Part model, mm, in its own coordinate system. Face numbers are marked on the shaded views. A direction names the side the tool comes from. Round coordinates to 2 decimals unless told otherwise and drop trailing zeros. Loops run counter-clockwise (first coordinate to the right, second up) from the corner with the lowest first, then second, coordinate; pieces in that order, holes last. Notation, with made-up numbers: M 86.25,33 L 123.25,33 A9 ccw 123.25,46 Z; hole C 61.5,-24.75 d7. An arc over 180 degrees is marked long. Put each result on its own line as item: value. Start each with the question number.
```python
from build123d import *

# Parameters (mm, degrees)
SKETCH1_W           = 10
SKETCH1_H           = 25.2
BOSS_EXTRUDE1_DEPTH = 4
SKETCH2_W           = 10
SKETCH2_H           = 3.2
SKETCH2_H_2         = 7.7
BOSS_EXTRUDE2_DEPTH = 7
SKETCH3_W           = 10
SKETCH3_H           = 4.5
BOSS_EXTRUDE3_DEPTH = 13
SKETCH4_R           = 3.1
CUT_EXTRUDE2_DEPTH  = 1
CHAMFER2_SIZE       = 1
CHAMFER3_SIZE       = 3


with BuildPart() as part:
    # Sketch1 → Boss-Extrude1 (new body)
    with BuildSketch(Plane.XY):
        with Locations((5, 12.6)):
            Rectangle(SKETCH1_W, SKETCH1_H)
    extrude(amount=BOSS_EXTRUDE1_DEPTH)

    # Sketch2 → Boss-Extrude2 (add)
    with BuildSketch(Plane(origin=(0, 0, 0), x_dir=(-1, 0, 0), z_dir=(0, 0, -1))):
        with Locations((-5, 23.6)):
            Rectangle(SKETCH2_W, SKETCH2_H)
        with Locations((-5, 12.85)):
            Rectangle(SKETCH2_W, SKETCH2_H_2)
    extrude(amount=BOSS_EXTRUDE2_DEPTH)

    # Sketch3 → Boss-Extrude3 (add)
    with BuildSketch(Plane.XY.offset(4)):
        with Locations((5, 2.25)):
            Rectangle(SKETCH3_W, SKETCH3_H)
    extrude(amount=BOSS_EXTRUDE3_DEPTH)

    # Sketch4 → Cut-Extrude2 (cut)
    with BuildSketch(Plane(origin=(0, 4.5, 0), x_dir=(1, 0, 0), z_dir=(0, 1, 0))):
        with Locations(Location((5, -9, 0), (0, 0, 270))):
            Circle(SKETCH4_R)
    extrude(amount=-CUT_EXTRUDE2_DEPTH, mode=Mode.SUBTRACT)

    # Chamfer2
    chamfer2_edges = [part.edges().sort_by_distance(p)[0] for p in [
        (5, 3.5, 5.9),
    ]]
    chamfer(chamfer2_edges, length=CHAMFER2_SIZE - 0.0001)  # a hair under: the kernel refuses the full size

    # Chamfer3
    chamfer3_edges = [part.edges().sort_by_distance(p)[0] for p in [
        (5, 25.2, 4),
        (5, 4.5, 17),
    ]]
    chamfer(chamfer3_edges, length=CHAMFER3_SIZE)


solid = part.part
```
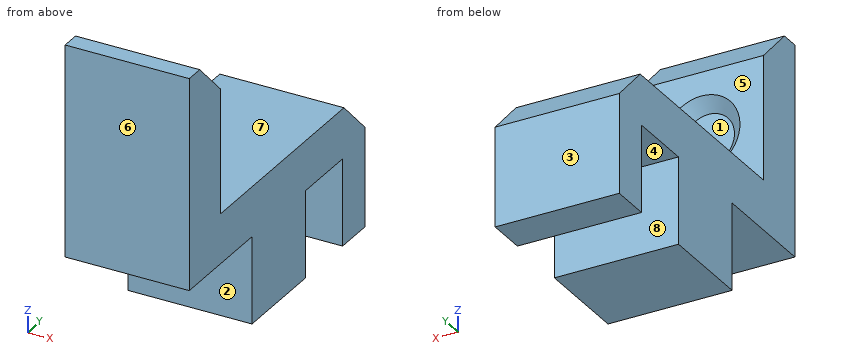
1. Wall check: L1, parallel to Y at x = 2, z = -4.75; L2, parallel to Y at x = 6.5, z = 9; L3, parallel to Z at x = 5, y = 4.55. Give the ranges that are in metal, low to high.
2. Mould opens along Y. For the marked faces 6, 7 and 8 say: released by +Y, released by -Y, zero draft, split by the parting line, or undercut.
3. Cut at D-D, the plane y = 2.25. Give the cut face in (x, z), and give its area (4 significant figures).
4. Drop flat-ended pins along their axis: pin 1 (4.5 mm diameter, centred on x = 4, z = 9, fed in from +Y); pin 2 (5 mm diameter, centred on x = 3.5, y = 17.5, fed in from +Z); pin 3 (2 mm diameter, centred on x = 4, z = -2.5, fed in from -Y). Give the stop position or say it passes through.
5. Which spindle directions (+Z, -Z, +X, -X, +Y, -Y) get a long thin tool onto all of the face, cutting with end or side? Do the marked faces 1, 2, 3, 4 and 5. Say none if no direction does.
6. Cut at A-A, the plane z = -3. Give the cut face in (x, y).
Results list:
1. L1: y = 9 to 16.7, 22 to 25.2
1. L2: y = 0 to 3.5
1. L3: z = 0 to 4
2. face 6: released by -Y
2. face 7: zero draft
2. face 8: undercut
3. outline: M 0,0 L 10,0 L 10,16.25 L 0,16.25 Z
3. area: 162.5 mm^2
4. pin 1: stops at y = 4.5
4. pin 2: stops at z = 4
4. pin 3: stops at y = 9
5. face 1: +Y
5. face 2: -Z, +X, -X, -Y
5. face 3: +Z, -Z, +X, -X, +Y
5. face 4: -Z, +X, -X
5. face 5: +Z, +X, -X, +Y
6. outline: M 0,9 L 10,9 L 10,16.7 L 0,16.7 Z; M 0,22 L 10,22 L 10,25.2 L 0,25.2 Z
